CAD build for the part. Positions are in the model's coordinates, mm. A direction names the side the tool comes from. Give positions to 0.01 mm unless a question says otherwise; leave off trailing zeros. Loops run counter-clockwise (first coordinate to the right, second up) from the corner with the lowest first, then second, coordinate; pieces in that order, holes last.
```python
from build123d import *

# Parameters (mm, degrees)
F1_DEPTH = 22


with BuildPart() as f1:
    # F0 (on Right) → F1 (new body)
    with BuildSketch(Plane.YZ):
        with BuildLine():
            Line((109.5, -2.0528280745), (109.5, 217.0326773285))
            Line((109.5, 217.0326773285), (-109.5, 217.0326773285))
            Line((-109.5, 217.0326773285), (-109.5, 168.5))
            add(Edge.make_bspline(
                [(-109.5, 168.5), (-27.7467335676, 133.469891204), (55.4140619779, 97.2245921781), (91.5, 41.4673226715)],
                knots=[0, 0, 0, 0, 0.3625910784, 0.3625910784, 0.3625910784, 0.3625910784], degree=3))
            add(Edge.make_bspline(
                [(91.5, 41.4673226715), (100.2961758102, 27.8761352961), (106.2952978286, 13.1256022765), (109.5, -2.0528280745)],
                knots=[0.3625910784, 0.3625910784, 0.3625910784, 0.3625910784, 0.4509749489, 0.4509749489, 0.4509749489, 0.4509749489], degree=3))
        make_face()
        with BuildLine():
            Line((109.5, -17.5326773285), (109.5, -2.0528280745))
            add(Edge.make_bspline(
                [(91.5, 41.4673226715), (100.2961758102, 27.8761352961), (106.2952978286, 13.1256022765), (109.5, -2.0528280745)],
                knots=[0.3625910784, 0.3625910784, 0.3625910784, 0.3625910784, 0.4509749489, 0.4509749489, 0.4509749489, 0.4509749489], degree=3))
            Line((91.5, 41.4673226715), (91.5, -28.5326773285))
            Line((91.5, -28.5326773285), (91.5, -98.5326773285))
            add(Edge.make_bspline(
                [(109.5, -54.8776239379), (106.2942898962, -70.0854206268), (100.2934101345, -84.8814155055), (91.5, -98.5326773285)],
                knots=[0.5523720652, 0.5523720652, 0.5523720652, 0.5523720652, 0.640815625, 0.640815625, 0.640815625, 0.640815625], degree=3))
            Line((109.5, -54.8776239379), (109.5, -39.5326773285))
            Line((109.5, -39.5326773285), (100.5, -39.5326773285))
            Line((100.5, -39.5326773285), (100.5, -17.5326773285))
            Line((100.5, -17.5326773285), (109.5, -17.5326773285))
        make_face()
        with BuildLine():
            Line((109.5, -217.0326773285), (109.5, -54.8776239379))
            add(Edge.make_bspline(
                [(109.5, -54.8776239379), (106.2942898962, -70.0854206268), (100.2934101345, -84.8814155055), (91.5, -98.5326773285)],
                knots=[0.5523720652, 0.5523720652, 0.5523720652, 0.5523720652, 0.640815625, 0.640815625, 0.640815625, 0.640815625], degree=3))
            add(Edge.make_bspline(
                [(91.5, -98.5326773285), (55.7884622504, -153.9727790026), (-25.9805742583, -190.5326773285), (-109.5, -217.0326773285)],
                knots=[0.640815625, 0.640815625, 0.640815625, 0.640815625, 1, 1, 1, 1], degree=3))
            Line((-109.5, -217.0326773285), (109.5, -217.0326773285))
        make_face()
    extrude(amount=F1_DEPTH)


solid = f1.part
```
1. Probe line 1 along Z through (x, y) = (16.5, -7); line 2 along Y through (x, z) = (11.75, -22); line 3 along Z through (x, y) = (7.75, -15.5). List the from-to ranges inside material, lowest first.
Responses:
line 1: z = -217.03 to -176.94, 121.12 to 217.03
line 2: y = 91.5 to 100.5
line 3: z = -217.03 to -181.05, 125.58 to 217.03
2. Tool access for faces 4 (the face through (22, 47, 99)), 5 (the face through (11, 105, -17.533)), 6 (the face through (11, 91.5, -28)): list every direction of +Z, -Z, +X, -X, +Y, -Y with a clear straight run to the whole face (end or side of a thin tool).
Responses:
face 4: +Z, -Z, +X, +Y, -Y
face 5: +X, -X, +Y
face 6: +X, -X, -Y
3. Drop flat-ended pins along their axis: pin 1 (12 mm diameter, centred on x = 16, z = -23.5, fed in from +Y); pin 2 (5 mm diameter, centred on x = 9.5, z = -139, fed in from -Y). Give the stop position or say it passes through.
Responses:
pin 1: stops at y = 109.5
pin 2: stops at y = 50.82
4. Saw through at B-B, the plane z = -23.5. List the corners of the cut face in (x, y), and give its area (3 significant figures).
Responses:
outline: (0, 91.5) - (22, 91.5) - (22, 100.5) - (0, 100.5) - close
area: 198 mm2
5. Pull direction Z, two halves, no side cores. Call faces 1 (the face through (11, 109.5, -130)), 2 (the face through (11, 100.5, -29)), 3 (the face through (11, -2, -217.033)): released by +Z, released by -Z, zero draft, split by the parting line, or undercut.
Responses:
face 1: zero draft
face 2: undercut
face 3: released by -Z
6. Saw through at A-A, the plane z = -71. List the corners of the cut face in (x, y).
Responses:
outline: (0, 91.5) - (22, 91.5) - (22, 109.5) - (0, 109.5) - close
